Build history of the part. All positions in model axes, mm. A direction names the side the tool comes from. Round coordinates to 2 decimals unless told otherwise and drop trailing zeros. Write each loop counter-clockwise with the first axis right and the second up, starting at its lowest first coordinate (ties: lowest second). Pieces come first, ordered by that corner, then holes.
Item 1: Band-saw the part on C-C, the plane z = 32. Write the cut outline in (x, y).
Item 2: 3-axis set-ups, long thin cutter, end or side, ignore diameter. For faces 4 (the flat face through (4.4, 2.4, 50.8)), 5 (the flat face through (0, 0, 16.669)), 6 (the flat face through (11, 0, 17.333)): which of +Z, -Z, +X, -X, +Y, -Y reach the whole face in a straight line?
Item 3: Mould opens along Y. For faces 1 (the flat face through (0, -2, 0)), 2 (the cylindrical face through (-0.34, 1.55, 8.22)), 3 (the conical face through (-1.43, 10.9, 0.45)) say: +Y half, -Y half, draft (parallel to the pull), parting line (faces both ways), or undercut.
Item 4: Wall check: probe 1 along Y at (x, z) = (0, 48); probe 2 along Z at (x, y) = (19.5, 10); probe 3 along Z at (x, y) = (-18, 1). Give the ranges that are in metal, low to high.
Item 5: Drop flat-ended pins along their axis: pin 1 Ø3 at (x, y) = (14.5, -2) entering from -Z; pin 2 Ø3 at (x, y) = (0, 0) entering from +Z (3 decimals); pin 3 Ø3 at (y, z) = (4, 38.5) entering from +X. Give the stop position or say it passes through.
```python
from build123d import *

# Parameters (mm, degrees)
F2_R     = 4.7625
F3_DEPTH = 9.525
F4_R     = 1.5875
F5_DEPTH = 16.66875


with BuildPart() as f1:
    # F0 (on Front) → F1 (revolve)
    with BuildSketch(Plane.XZ):
        with BuildLine():
            Line((0, 50.8), (0, 0))
            Line((0, 0), (10.261248, 0))
            Line((10.261248, 0), (21.929258, 7.154912))
            ThreePointArc((21.929258, 7.154912), (24.1506, 9.46627), (24.959791, 12.568196))
            Line((24.959791, 12.568196), (24.959791, 17.333189))
            Line((24.959791, 17.333189), (10.261248, 17.333189))
            Line((10.261248, 17.333189), (10.261248, 50.8))
            Line((10.261248, 50.8), (0, 50.8))
        make_face()
    revolve(axis=Axis((0, 0, 25.4), (0, 0, 1)))

    # F2 (on face) → F3 (cut)
    with BuildSketch(Plane.XY.offset(50.8)):
        Circle(F2_R)
    extrude(amount=-F3_DEPTH, mode=Mode.SUBTRACT)

    # F4 (on face) → F5 (cut)
    with BuildSketch(Plane(origin=(0, 0, 0), x_dir=(1, 0, 0), z_dir=(0, 0, -1))):
        Circle(F4_R)
    extrude(amount=-F5_DEPTH, mode=Mode.SUBTRACT)


solid = f1.part
```
Results:
1. outline: circle Ø20.52 at (0, 0)
2. face 4: +Z, +X, -X, +Y, -Y
2. face 5: -Z
2. face 6: +Z
3. face 1: draft
3. face 2: undercut
3. face 3: parting line
4. probe 1: y = -10.26 to -4.76, 4.76 to 10.26
4. probe 2: z = 7.15 to 17.33
4. probe 3: z = 4.76 to 17.33
5. pin 1: stops at z = 1.76
5. pin 2: stops at z = 41.275
5. pin 3: stops at x = 9.95
